Source: CAD feature listing. Evaluate the final solid. Frame: model axes, mm. Face numbers are marked on the shaded views. A direction names the side the tool comes from. Round coordinates to 2 decimals unless told otherwise and drop trailing zeros. Loops run counter-clockwise (first coordinate to the right, second up) from the corner with the lowest first, then second, coordinate; pieces in that order, holes last. Notation, with made-up numbers: M -9,39.25 L 44,39.25 A16 cw 44,52.25 Z; hole C -24.75,-13.5 d4. An arc over 180 degrees is marked long. One line per item, written item: value.
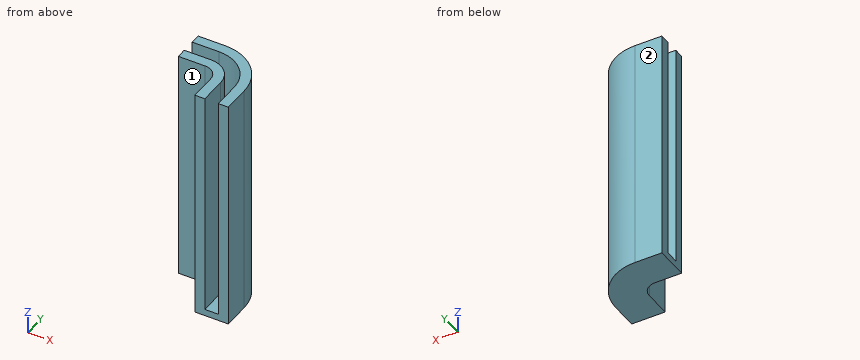
from build123d import *

# Parameters (mm, degrees)
F2_DEPTH = 1
F3_DEPTH = 35


# Not quite as in the source:
# - a feature names something its author has since deleted; it is built from what else it names


with BuildPart() as f2:
    # F1 (on Top) → F2 (new body)
    with BuildSketch(Plane.XY):
        with BuildLine():
            Line((-4, 5.5), (-4, 3.7749172176))
            ThreePointArc((-4, 3.7749172176), (-2.1780674121, 5.0503487353), (0, 5.5))
            Line((0, 5.5), (-4, 5.5))
        make_face()
        with BuildLine():
            ThreePointArc((5.5, 0), (5.0503487353, -2.1780674121), (3.7749172176, -4))
            Line((3.7749172176, -4), (5.5, -4))
            Line((5.5, -4), (5.5, 0))
        make_face()
        with BuildLine():
            Line((-4, 7), (-4, 5.7445626465))
            ThreePointArc((-4, 5.7445626465), (-2.0961943462, 6.6787700412), (0, 7))
            Line((0, 7), (-4, 7))
        make_face()
        with BuildLine():
            ThreePointArc((7, 0), (6.6787700412, -2.0961943462), (5.7445626465, -4))
            Line((5.7445626465, -4), (7, -4))
            Line((7, -4), (7, 0))
        make_face()
        with BuildLine():
            Line((-4, 2), (-2.8722813233, 2))
            ThreePointArc((-2.8722813233, 2), (-1.6201851746, 3.1024184115), (0, 3.5))
            Line((0, 3.5), (-4, 3.5))
            Line((-4, 3.5), (-4, 2))
        make_face()
        with BuildLine():
            ThreePointArc((3.5, 0), (3.1024184115, -1.6201851746), (2, -2.8722813233))
            Line((2, -2.8722813233), (2, -4))
            Line((2, -4), (3.5, -4))
            Line((3.5, -4), (3.5, 0))
        make_face()
        with BuildLine():
            ThreePointArc((0, 2), (1.4142135624, 1.4142135624), (2, 0))
            Line((2, 0), (2, -2.8722813233))
            ThreePointArc((2, -2.8722813233), (3.1024184115, -1.6201851746), (3.5, 0))
            ThreePointArc((3.5, 0), (2.4748737342, 2.4748737342), (0, 3.5))
            ThreePointArc((0, 3.5), (-1.6201851746, 3.1024184115), (-2.8722813233, 2))
            Line((-2.8722813233, 2), (0, 2))
        make_face()
        with BuildLine():
            ThreePointArc((0, 3.5), (2.4748737342, 2.4748737342), (3.5, 0))
            Line((3.5, 0), (3.5, -4))
            Line((3.5, -4), (3.7749172176, -4))
            ThreePointArc((3.7749172176, -4), (5.0503487353, -2.1780674121), (5.5, 0))
            ThreePointArc((5.5, 0), (3.8890872965, 3.8890872965), (0, 5.5))
            ThreePointArc((0, 5.5), (-2.1780674121, 5.0503487353), (-4, 3.7749172176))
            Line((-4, 3.7749172176), (-4, 3.5))
            Line((-4, 3.5), (0, 3.5))
        make_face()
        with BuildLine():
            ThreePointArc((0, 5.5), (3.8890872965, 3.8890872965), (5.5, 0))
            Line((5.5, 0), (5.5, -4))
            Line((5.5, -4), (5.7445626465, -4))
            ThreePointArc((5.7445626465, -4), (6.6787700412, -2.0961943462), (7, 0))
            ThreePointArc((7, 0), (4.9497474683, 4.9497474683), (0, 7))
            ThreePointArc((0, 7), (-2.0961943462, 6.6787700412), (-4, 5.7445626465))
            Line((-4, 5.7445626465), (-4, 5.5))
            Line((-4, 5.5), (0, 5.5))
        make_face()
    extrude(amount=F2_DEPTH)

    # F1 (on Top) → F3 (join)
    with BuildSketch(Plane.XY):
        with BuildLine():
            ThreePointArc((0, 5.5), (3.8890872965, 3.8890872965), (5.5, 0))
            Line((5.5, 0), (5.5, -4))
            Line((5.5, -4), (5.7445626465, -4))
            ThreePointArc((5.7445626465, -4), (6.6787700412, -2.0961943462), (7, 0))
            ThreePointArc((7, 0), (4.9497474683, 4.9497474683), (0, 7))
            ThreePointArc((0, 7), (-2.0961943462, 6.6787700412), (-4, 5.7445626465))
            Line((-4, 5.7445626465), (-4, 5.5))
            Line((-4, 5.5), (0, 5.5))
        make_face()
        with BuildLine():
            Line((-4, 7), (-4, 5.7445626465))
            ThreePointArc((-4, 5.7445626465), (-2.0961943462, 6.6787700412), (0, 7))
            Line((0, 7), (-4, 7))
        make_face()
        with BuildLine():
            ThreePointArc((7, 0), (6.6787700412, -2.0961943462), (5.7445626465, -4))
            Line((5.7445626465, -4), (7, -4))
            Line((7, -4), (7, 0))
        make_face()
        with BuildLine():
            ThreePointArc((3.5, 0), (3.1024184115, -1.6201851746), (2, -2.8722813233))
            Line((2, -2.8722813233), (2, -4))
            Line((2, -4), (3.5, -4))
            Line((3.5, -4), (3.5, 0))
        make_face()
        with BuildLine():
            ThreePointArc((0, 2), (1.4142135624, 1.4142135624), (2, 0))
            Line((2, 0), (2, -2.8722813233))
            ThreePointArc((2, -2.8722813233), (3.1024184115, -1.6201851746), (3.5, 0))
            ThreePointArc((3.5, 0), (2.4748737342, 2.4748737342), (0, 3.5))
            ThreePointArc((0, 3.5), (-1.6201851746, 3.1024184115), (-2.8722813233, 2))
            Line((-2.8722813233, 2), (0, 2))
        make_face()
        with BuildLine():
            Line((-4, 2), (-2.8722813233, 2))
            ThreePointArc((-2.8722813233, 2), (-1.6201851746, 3.1024184115), (0, 3.5))
            Line((0, 3.5), (-4, 3.5))
            Line((-4, 3.5), (-4, 2))
        make_face()
    extrude(amount=F3_DEPTH)


solid = f2.part
1. Pin query (flat end, axial travel): pin 1 (3 mm diameter, centred on y = -2.5, z = 20.5, fed in from -X); pin 2 (1.2 mm diameter, centred on x = -2.5, z = 10.5, fed in from -Y); pin 3 (3 mm diameter, centred on x = -0.5, z = 23, fed in from -Y). Return the tip coordinate at first contact, or that it passes through.
Report:
pin 1: stops at x = 2
pin 2: stops at y = 2
pin 3: stops at y = 1.73
2. Reachability of the marked faces 1 and 2 from +Z, -Z, +X, -X, +Y, -Y: full face, straight path, thin tool, end or side. Return the list, or none.
Report:
face 1: +Z, -Z, -X, -Y
face 2: +Z, -Z, +X, -X, +Y
3. Section query B-B (x = -1.25). Return the cut outline in (y, z), and give its area (3 significant figures).
Report:
outline: M 2,0 L 7,0 L 7,35 L 5.5,35 L 5.5,1 L 3.5,1 L 3.5,35 L 2,35 Z
area: 107 mm2
4. Section query A-A (z = 31). Return the cut outline in (x, y), and give its area (3 significant figures).
Report:
outline: M -4,2 L 0,2 A2 cw 2,0 L 2,-4 L 3.5,-4 L 3.5,0 A3.5 ccw 0,3.5 L -4,3.5 Z; M -4,5.5 L 0,5.5 A5.5 cw 5.5,0 L 5.5,-4 L 7,-4 L 7,0 A7 ccw 0,7 L -4,7 Z
area: 45.2 mm2
5. Ray query, line 1 (X direction, y = -0.5, z = 17.5); line 2 (X direction, y = 1.25, z = 30). Return the intervals inside material, ascending. Write a range as [from, to].
Report:
line 1: x = [2, 3.5], [5.5, 7]
line 2: x = [1.56, 3.27], [5.36, 6.89]
6. Section query D-D (x = 4.75). Return the cut outline in (y, z).
Report:
outline: M -4,0 L 5.14,0 L 5.14,35 L 2.77,35 L 2.77,1 L -4,1 Z
